```python
from build123d import *

# Parameters (mm, degrees)
SKETCH1_W           = 33
SKETCH1_H           = 11
SKETCH1_W_2         = 30
SKETCH1_H_2         = 8
BOSS_EXTRUDE1_DEPTH = 8
SKETCH1_6_W         = 30
SKETCH1_6_H         = 8
CUT_EXTRUDE1_DEPTH  = 8
CUT_EXTRUDE1_TAPER  = 17
CUT_EXTRUDE3_REACH  = 23.383
SKETCH3_R           = 0.8
BOSS_EXTRUDE6_DEPTH = 2
CUT_EXTRUDE4_DEPTH  = 23.209232315
CUT_EXTRUDE5_START  = -5.955717
SKETCH5_R           = 3.375
CUT_EXTRUDE5_DEPTH  = 7.955717
SKETCH6_W           = 30.5
SKETCH6_H           = 8.5
CUT_EXTRUDE6_DEPTH  = 2.25
FILLET1_R           = 1


with BuildPart() as part:
    # Sketch1 → Boss-Extrude1 (new body)
    # profile 1 of 2: a face of its own
    with BuildSketch(Plane(origin=(0, 0, 0), x_dir=(1, 0, 0), z_dir=(0, 1, 0))):
        Rectangle(SKETCH1_W, SKETCH1_H)
        Rectangle(SKETCH1_W_2, SKETCH1_H_2, mode=Mode.SUBTRACT)
    # profile 2 of 2: a face of its own
    with BuildSketch(Plane(origin=(0, 0, 0), x_dir=(1, 0, 0), z_dir=(0, 1, 0))):
        Rectangle(SKETCH1_W_2, SKETCH1_H_2)
    extrude(amount=BOSS_EXTRUDE1_DEPTH)

    # Sketch1<6> → Cut-Extrude1 (cut)
    with BuildSketch(Plane(origin=(0, 0, 0), x_dir=(1, 0, 0), z_dir=(0, 1, 0))):
        Rectangle(SKETCH1_6_W, SKETCH1_6_H)
    extrude(amount=CUT_EXTRUDE1_DEPTH, taper=CUT_EXTRUDE1_TAPER, mode=Mode.SUBTRACT)

    # Cut-Extrude3: up to this plane
    cut_extrude3_end = Plane(origin=(0, 0, 4), z_dir=(0, 0.2923717047227373, 0.9563047559630353))
    # Sketch3 → Cut-Extrude3 (cut, up to the surface)
    with BuildSketch(Plane.XY.offset(5.5), mode=Mode.PRIVATE) as cut_extrude3_sk1:
        with Locations((-12.5, 4)):
            Circle(SKETCH3_R)
    cut_extrude3_tool1 = split(extrude(cut_extrude3_sk1.sketch, amount=-CUT_EXTRUDE3_REACH, mode=Mode.PRIVATE), bisect_by=cut_extrude3_end, keep=Keep.BOTH, mode=Mode.PRIVATE)
    # Sketch3 → Cut-Extrude3 (cut, up to the surface)
    with BuildSketch(Plane.XY.offset(5.5), mode=Mode.PRIVATE) as cut_extrude3_sk2:
        with Locations((12.5, 4)):
            Circle(SKETCH3_R)
    cut_extrude3_tool2 = split(extrude(cut_extrude3_sk2.sketch, amount=-CUT_EXTRUDE3_REACH, mode=Mode.PRIVATE), bisect_by=cut_extrude3_end, keep=Keep.BOTH, mode=Mode.PRIVATE)
    cut_extrude3 = cut_extrude3_tool1.solids().sort_by_distance((-12.5, 4, 5.5))[0] + cut_extrude3_tool2.solids().sort_by_distance((12.5, 4, 5.5))[0]
    add(cut_extrude3, mode=Mode.SUBTRACT)

    # Mirror1: Cut-Extrude3 across plane
    add(cut_extrude3.mirror(Plane.XY), mode=Mode.SUBTRACT)

    # Sketch2<6> → Boss-Extrude6 (add)
    with BuildSketch(Plane(origin=(0, 8, 0), x_dir=(1, 0, 0), z_dir=(0, 1, 0))):
        with BuildLine():
            Line((3.799705909, -3.054154548), (14.054154548, -3.054154548))
            Line((14.054154548, -3.054154548), (14.054154548, 3.054154548))
            Line((14.054154548, 3.054154548), (3.799705909, 3.054154548))
            ThreePointArc((3.799705909, 3.054154548), (0, 4.875), (-3.799705909, 3.054154548))
            Line((-3.799705909, 3.054154548), (-14.054154548, 3.054154548))
            Line((-14.054154548, 3.054154548), (-14.054154548, -3.054154548))
            Line((-14.054154548, -3.054154548), (-3.799705909, -3.054154548))
            ThreePointArc((-3.799705909, -3.054154548), (0, -4.875), (3.799705909, -3.054154548))
        make_face()
        with BuildLine():
            ThreePointArc((2.995868595, 1.554154548), (3.375, 0), (2.995868595, -1.554154548))
            Line((2.995868595, -1.554154548), (1.626992206, -1.554154548))
            ThreePointArc((1.626992206, -1.554154548), (0, -2.25), (-1.626992206, -1.554154548))
            Line((-1.626992206, -1.554154548), (-2.995868595, -1.554154548))
            ThreePointArc((-2.995868595, -1.554154548), (-3.375, 0), (-2.995868595, 1.554154548))
            Line((-2.995868595, 1.554154548), (-1.626992206, 1.554154548))
            ThreePointArc((-1.626992206, 1.554154548), (0, 2.25), (1.626992206, 1.554154548))
            Line((1.626992206, 1.554154548), (2.995868595, 1.554154548))
        make_face(mode=Mode.SUBTRACT)
    extrude(amount=BOSS_EXTRUDE6_DEPTH)

    # Sketch4 → Cut-Extrude4 (cut, through all)
    with BuildSketch(Plane.XY.offset(5.5)):
        Polygon((-16.5, 0), (-14.054154548, 8), (-16.5, 8), align=None)
        Polygon((16.5, 0), (14.054154548, 8), (16.5, 8), align=None)
    extrude(amount=-CUT_EXTRUDE4_DEPTH, mode=Mode.SUBTRACT)

    # Sketch5 → Cut-Extrude5 (cut)
    with BuildSketch(Plane(origin=(0, 8, 0), x_dir=(1, 0, 0), z_dir=(0, 1, 0)).offset(CUT_EXTRUDE5_START)):
        with Locations(Location((0, 0, 0), (0, 0, 27.418746095))):
            Circle(SKETCH5_R)
    extrude(amount=CUT_EXTRUDE5_DEPTH, mode=Mode.SUBTRACT)

    # Sketch6 → Cut-Extrude6 (cut)
    with BuildSketch(Plane.XZ):
        Rectangle(SKETCH6_W, SKETCH6_H)
    extrude(amount=-CUT_EXTRUDE6_DEPTH, mode=Mode.SUBTRACT)

    # Fillet1
    fillet1_edges = [part.edges().sort_by_distance(p)[0] for p in [
        (8.926930229, 8, 3.054154548),
        (-8.926930229, 8, -3.054154548),
        (0, 8, -4.875),
        (-8.926930229, 8, 3.054154548),
        (0, 8, 4.875),
        (8.926930229, 8, -3.054154548),
    ]]
    fillet(fillet1_edges, radius=FILLET1_R)


solid = part.part
```
Could you check a few things on this model? Use its own coordinates, in mm. A direction names the side the tool comes from. Give positions to 0.01 mm unless a question says otherwise; leave off trailing zeros. Order: outer loops, then holes, each group sorted by start corner. A loop starts at its lowest first (then second) coordinate and runs counter-clockwise, first axis right, second up.
Q1. If I drill on line 1 along X through (y, z) = (4, -4.45); line 2 along Y through (x, z) = (-12.5, 3.95); line 3 along Z through (x, y) = (-9, 2), over which ranges is the centre line in solid material (lowest first)?
Q2. Suppose I cut it at A-A, the plane y = 1.75. Write out the boundary of the cut face in (x, z).
Q3. I'm going to push flat-ended pins straight in: P1, Ø1.1, axis at y = 1.5, z = -0.5, coming from the +X side; P2, Ø0.9, axis at x = 6, z = 0.5, coming from the -Y side; P3, Ø1, axis at y = 6, z = 3, coming from the +X side. Where does each tip first touch, or does it pass through?
Q4. For faces 5 (the flat face through (8, 8, 0)), 6 (the flat face through (8, 8, 5)), 7 (the cylindrical face through (0.061, 9.441, -4.875)), 8 (the flat face through (-9, 9.5, 3.054)), 9 (the flat face through (-8, 8, -5)), which set-ups out of +Z, -Z, +X, -X, +Y, -Y let a thin tool reach every point of the face, with its end or its side?
Q5. Suppose I cut it at B-B, the plane y = 4. Count the separate pieces of the cut face and the enclosed holes in it, and give its area (3 significant figures).
Q6. We'd pull the mould along X, two halves only. Please class faces 1 (the flat face through (15.294, 3.944, 0.077)), 2 (the cylindrical face through (12.396, 4.793, -4.013)), 3 (the cylindrical face through (-12.604, 4.793, 4.013)), 4 (the flat face through (0, 4, -5.5)): +X half, -X half, draft (parallel to the pull), parting line (faces both ways), or undercut.
Solution:
1. line 1: x = -15.28 to -13.3, -11.7 to 11.7, 13.3 to 15.28
1. line 2: y = 2.25 to 3.2, 4.8 to 8.01
1. line 3: z = -5.5 to -4.25, 4.25 to 5.5
2. outline: (-15.96, -5.5) - (15.96, -5.5) - (15.96, 5.5) - (-15.96, 5.5) - close; hole (-15.25, -4.25) - (15.25, -4.25) - (15.25, 4.25) - (-15.25, 4.25) - close
3. P1: stops at x = 16.21
3. P2: stops at y = 8
3. P3: stops at x = 14.82
4. face 5: -Y
4. face 6: +Z, +X, +Y
4. face 7: -Z, +Y
4. face 8: +Z, -X, +Y
4. face 9: -Z, -X, +Y
5. separate pieces: 4
5. enclosed holes: 0
5. area: 163 mm2
6. face 1: +X half
6. face 2: undercut
6. face 3: undercut
6. face 4: draft
